```python
from build123d import *

# Parameters (mm, degrees)
SKETCH1_R           = 185
BOSS_EXTRUDE1_DEPTH = 350
FILLET1_R           = 30
BOSS_EXTRUDE2_DEPTH = 100
SKETCH3_R           = 12.5
BOSS_EXTRUDE3_DEPTH = 60


with BuildPart() as part:
    # Sketch1 → Boss-Extrude1 (new, symmetric)
    with BuildSketch(Plane.XY):
        Circle(SKETCH1_R)
    extrude(amount=BOSS_EXTRUDE1_DEPTH, both=True)

    # Fillet1
    fillet1_edges = [part.edges().sort_by_distance(p)[0] for p in [
        (-185, 0, -350),
        (-185, 0, 350),
    ]]
    fillet(fillet1_edges, radius=FILLET1_R)

    # Sketch2 → Boss-Extrude2 (add, symmetric)
    with BuildSketch(Plane.XY):
        Polygon((0, 0), (200, -200), (-200, -200), align=None)
    extrude(amount=BOSS_EXTRUDE2_DEPTH, both=True)

    # Sketch3 → Boss-Extrude3 (add)
    with BuildSketch(Plane.XY.offset(350)):
        Circle(SKETCH3_R)
    extrude(amount=BOSS_EXTRUDE3_DEPTH)


solid = part.part
```
Can you work these out from the model? Positions are in its coordinate system, mm. A direction names the side the tool comes from. Coordinates: 2 decimals unless noted, no trailing zeros. Order: outer loops, then holes, each group sorted by start corner. A loop starts at its lowest first (then second) coordinate and runs counter-clockwise, first axis right, second up. Notation, with made-up numbers: (32, 10.5) -> (64, 10.5) arc R25 ccw to (64, 38.5) -> close; hole circle Ø10 at (-14, -4.75). An arc over 180 degrees is marked (long way). Write each question's results on one line, items separated by ' | '.
Item 1: I want a section at C-C, the plane z = -181.5. Write out the boundary of the cut face in (x, y), then the cut area to 3 significant figures.
Results are:
outline: circle Ø370 at (0, 0) | area: 108,000 mm²
Item 2: I want a section at B-B, the plane x = 0. Write out the boundary of the cut face in (y, z).
Results are:
outline: (-200, -100) -> (-185, -100) -> (-185, -320) arc R30 ccw to (-155, -350) -> (155, -350) arc R30 ccw to (185, -320) -> (185, 320) arc R30 ccw to (155, 350) -> (12.5, 350) -> (12.5, 410) -> (-12.5, 410) -> (-12.5, 350) -> (-155, 350) arc R30 ccw to (-185, 320) -> (-185, 100) -> (-200, 100) -> close
Item 3: If we mould it in two halves opening along Y, with no side actions, what happens to faces 4 (the face through (-2, -32, 350)), 5 (the face through (11.923, 3.755, 379.58)), 6 (the face through (-166, -166, 1))? For each: +Y half, -Y half, draft (parallel to the pull), parting line (faces both ways), or undercut.
Results are:
face 4: draft | face 5: parting line | face 6: undercut
Item 4: I'm going to push flat-ended pins straight in: pin 1 Ø2 at (x, z) = (48.5, -221.5) entering from -Y; pin 2 Ø4 at (x, z) = (-19, -0.5) entering from +Y; pin 3 Ø5 at (x, z) = (119, -54.5) entering from +Y. Where does each tip first touch, or does it pass through?
Results are:
pin 1: y = -178.8 | pin 2: y = 184.22 | pin 3: y = 143.71
Item 5: I want a section at A-A, the plane y = 0. Write out the boundary of the cut face in (x, z), then the cut area to 3 significant figures.
Results are:
outline: (-185, -320) arc R30 ccw to (-155, -350) -> (155, -350) arc R30 ccw to (185, -320) -> (185, 320) arc R30 ccw to (155, 350) -> (12.5, 350) -> (12.5, 410) -> (-12.5, 410) -> (-12.5, 350) -> (-155, 350) arc R30 ccw to (-185, 320) -> close | area: 260,000 mm²
Item 6: I want a section at D-D, the plane z = 29.5. Write out the boundary of the cut face in (x, y), then the cut area to 3 significant figures.
Results are:
outline: (-200, -200) -> (200, -200) -> (130.81, -130.81) arc R185 ccw (long way) to (-130.81, -130.81) -> close | area: 121,000 mm²
Item 7: Which directions (+Z, -Z, +X, -X, +Y, -Y) give clear straight access to the entire face, cutting with the end or side of a thin tool? Please do faces 1 (the face through (3, -188, 100)), 2 (the face through (165, -165, 1)), 3 (the face through (3, -188, -100)).
Results are:
face 1: +Z, -Y | face 2: +Z, -Z, +X | face 3: -Z, -Y
Item 8: If I drill on line 1 along Z through (x, y) = (-149.5, 45); line 2 along Y through (x, z) = (43, 278); line 3 along Y through (x, z) = (-52.5, 265), over which ranges is the centre line in solid material (lowest first)?
Results are:
line 1: -349.98 to 349.98 | line 2: -179.93 to 179.93 | line 3: -177.39 to 177.39
